The model under review builds one solid part; all positions refer to its coordinate system, in mm. A direction names the side the tool comes from. Give positions to 0.01 mm unless a question says otherwise; leave off trailing zeros. Order: outer loops, then holes, each group sorted by start corner. A loop starts at its lowest first (then second) coordinate and runs counter-clockwise, first axis right, second up. Notation, with made-up numbers: (36, 68.25) -> (90, 68.25) arc R27 ccw to (90, 104.25) -> close; hole circle Ø8 at (15.5, 79). An arc over 180 degrees is marked (long way). Use one line per item in the form item = value.
```python
from build123d import *

# Parameters (mm, degrees)
BASE_FLANGE2_DEPTH         = 3.175
SKETCHED_START             = -176
SKETCHED_BEND3_OUTLINE_W   = 3.175
SKETCHED_BEND3_OUTLINE_H   = 145
SKETCHED_BEND3_DEPTH       = 112.825
SKETCHED_START_2           = 63.175
SKETCHED_BEND3_2_OUTLINE_W = 3.175
SKETCHED_BEND3_2_OUTLINE_H = 145
SKETCHED_BEND3_2_DEPTH     = 112.825
SKETCHED_START_3           = -62.794557784
SKETCHED_BEND3_3_DEPTH     = 2.794557784
SKETCHED_START_4           = 60
SKETCHED_BEND3_4_DEPTH     = 2.794557784
SKETCHED_START_5           = -63.175
SKETCHED_BEND3_5_DEPTH     = 3.9116
SKETCHED_START_6           = 59.2634
SKETCHED_BEND3_6_DEPTH     = 3.9116
SKETCHED_START_7           = -81
SKETCHED_BEND3_7_DEPTH     = 147


with BuildPart() as part:
    # Base-Flange2: sheet metal written as solids
    # Sketch1 → Base-Flange2 (new body)
    with BuildSketch(Plane(origin=(0, 0, 0), x_dir=(1, 0, 0), z_dir=(0, 1, 0))):
        with BuildLine():
            Line((-95, 80), (95, 80))
            Line((95, 80), (138.886329547, 58.22868679))
            ThreePointArc((138.886329547, 58.22868679), (173.284534609, -14.834678268), (110, -65))
            Line((110, -65), (-110, -65))
            ThreePointArc((-110, -65), (-173.284534609, -14.834678268), (-138.886329547, 58.22868679))
            Line((-138.886329547, 58.22868679), (-95, 80))
        make_face()
        with BuildLine():
            Line((100, -15), (120, -15))
            ThreePointArc((120, -15), (123.535533906, -13.535533906), (125, -10))
            Line((125, -10), (125, 10))
            ThreePointArc((125, 10), (123.535533906, 13.535533906), (120, 15))
            Line((120, 15), (100, 15))
            ThreePointArc((100, 15), (96.464466094, 13.535533906), (95, 10))
            Line((95, 10), (95, -10))
            ThreePointArc((95, -10), (96.464466094, -13.535533906), (100, -15))
        make_face(mode=Mode.SUBTRACT)
        with BuildLine():
            Line((-100, -15), (-120, -15))
            ThreePointArc((-120, -15), (-123.535533906, -13.535533906), (-125, -10))
            Line((-125, -10), (-125, 10))
            ThreePointArc((-125, 10), (-123.535533906, 13.535533906), (-120, 15))
            Line((-120, 15), (-100, 15))
            ThreePointArc((-100, 15), (-96.464466094, 13.535533906), (-95, 10))
            Line((-95, 10), (-95, -10))
            ThreePointArc((-95, -10), (-96.464466094, -13.535533906), (-100, -15))
        make_face(mode=Mode.SUBTRACT)
    extrude(amount=-BASE_FLANGE2_DEPTH)

    # Sketched Bend3: read off the stored shape, not the designer's step
    # Sketched Bend3 outline → Sketched Bend3 (cut)
    with BuildSketch(Plane.YZ.offset(SKETCHED_START)):
        with Locations((-1.5875, -7.5)):
            Rectangle(SKETCHED_BEND3_OUTLINE_W, SKETCHED_BEND3_OUTLINE_H)
    extrude(amount=SKETCHED_BEND3_DEPTH, mode=Mode.SUBTRACT)

    # Sketched Bend3 2 outline → Sketched Bend3 2 (cut)
    with BuildSketch(Plane.YZ.offset(SKETCHED_START_2)):
        with Locations((-1.5875, -7.5)):
            Rectangle(SKETCHED_BEND3_2_OUTLINE_W, SKETCHED_BEND3_2_OUTLINE_H)
    extrude(amount=SKETCHED_BEND3_2_DEPTH, mode=Mode.SUBTRACT)

    # Sketched Bend3 3 outline → Sketched Bend3 3 (add)
    with BuildSketch(Plane.YZ.offset(SKETCHED_START_3)):
        with BuildLine():
            Line((47.822512257, 65), (0, 65))
            Line((0, 65), (0, -80))
            Line((0, -80), (32.822512257, -80))
            Line((32.822512257, -80), (76.708841804, -58.22868679))
            ThreePointArc((76.708841804, -58.22868679), (111.107046866, 14.834678268), (47.822512257, 65))
        make_face()
        with BuildLine():
            ThreePointArc((62.822512257, -10), (61.358046163, -13.535533906), (57.822512257, -15))
            Line((57.822512257, -15), (37.822512257, -15))
            ThreePointArc((37.822512257, -15), (34.286978351, -13.535533906), (32.822512257, -10))
            Line((32.822512257, -10), (32.822512257, 10))
            ThreePointArc((32.822512257, 10), (34.286978351, 13.535533906), (37.822512257, 15))
            Line((37.822512257, 15), (57.822512257, 15))
            ThreePointArc((57.822512257, 15), (61.358046163, 13.535533906), (62.822512257, 10))
            Line((62.822512257, 10), (62.822512257, -10))
        make_face(mode=Mode.SUBTRACT)
    extrude(amount=SKETCHED_BEND3_3_DEPTH)

    # Sketched Bend3 4 outline → Sketched Bend3 4 (add)
    with BuildSketch(Plane.YZ.offset(SKETCHED_START_4)):
        with BuildLine():
            Line((47.822512257, 65), (0, 65))
            Line((0, 65), (0, -80))
            Line((0, -80), (32.822512257, -80))
            Line((32.822512257, -80), (76.708841804, -58.22868679))
            ThreePointArc((76.708841804, -58.22868679), (111.107046866, 14.834678268), (47.822512257, 65))
        make_face()
        with BuildLine():
            ThreePointArc((62.822512257, -10), (61.358046163, -13.535533906), (57.822512257, -15))
            Line((57.822512257, -15), (37.822512257, -15))
            ThreePointArc((37.822512257, -15), (34.286978351, -13.535533906), (32.822512257, -10))
            Line((32.822512257, -10), (32.822512257, 10))
            ThreePointArc((32.822512257, 10), (34.286978351, 13.535533906), (37.822512257, 15))
            Line((37.822512257, 15), (57.822512257, 15))
            ThreePointArc((57.822512257, 15), (61.358046163, 13.535533906), (62.822512257, 10))
            Line((62.822512257, 10), (62.822512257, -10))
        make_face(mode=Mode.SUBTRACT)
    extrude(amount=SKETCHED_BEND3_4_DEPTH)

    # Sketched Bend3 5 outline → Sketched Bend3 5 (add)
    with BuildSketch(Plane.YZ.offset(SKETCHED_START_5)):
        with BuildLine():
            ThreePointArc((76.708841804, -58.22868679), (111.107046866, 14.834678268), (47.822512257, 65))
            Line((47.822512257, 65), (0, 65))
            Line((0, 65), (0, -80))
            Line((0, -80), (32.822512257, -80))
            Line((32.822512257, -80), (76.708841804, -58.22868679))
        make_face()
        with BuildLine():
            ThreePointArc((62.822512257, -10), (61.358046163, -13.535533906), (57.822512257, -15))
            Line((57.822512257, -15), (37.822512257, -15))
            ThreePointArc((37.822512257, -15), (34.286978351, -13.535533906), (32.822512257, -10))
            Line((32.822512257, -10), (32.822512257, 10))
            ThreePointArc((32.822512257, 10), (34.286978351, 13.535533906), (37.822512257, 15))
            Line((37.822512257, 15), (57.822512257, 15))
            ThreePointArc((57.822512257, 15), (61.358046163, 13.535533906), (62.822512257, 10))
            Line((62.822512257, 10), (62.822512257, -10))
        make_face(mode=Mode.SUBTRACT)
    extrude(amount=SKETCHED_BEND3_5_DEPTH)

    # Sketched Bend3 6 outline → Sketched Bend3 6 (add)
    with BuildSketch(Plane.YZ.offset(SKETCHED_START_6)):
        with BuildLine():
            ThreePointArc((76.708841804, -58.22868679), (111.107046866, 14.834678268), (47.822512257, 65))
            Line((47.822512257, 65), (0, 65))
            Line((0, 65), (0, -80))
            Line((0, -80), (32.822512257, -80))
            Line((32.822512257, -80), (76.708841804, -58.22868679))
        make_face()
        with BuildLine():
            ThreePointArc((62.822512257, -10), (61.358046163, -13.535533906), (57.822512257, -15))
            Line((57.822512257, -15), (37.822512257, -15))
            ThreePointArc((37.822512257, -15), (34.286978351, -13.535533906), (32.822512257, -10))
            Line((32.822512257, -10), (32.822512257, 10))
            ThreePointArc((32.822512257, 10), (34.286978351, 13.535533906), (37.822512257, 15))
            Line((37.822512257, 15), (57.822512257, 15))
            ThreePointArc((57.822512257, 15), (61.358046163, 13.535533906), (62.822512257, 10))
            Line((62.822512257, 10), (62.822512257, -10))
        make_face(mode=Mode.SUBTRACT)
    extrude(amount=SKETCHED_BEND3_6_DEPTH)

    # Sketched Bend3 7 outline → Sketched Bend3 7 (cut)
    with BuildSketch(Plane.XY.offset(SKETCHED_START_7)):
        with BuildLine():
            Line((-65, -3.175000031), (-59.2634, -3.175))
            ThreePointArc((-59.2634, -3.175), (-62.029318885, -2.029318885), (-63.175, 0.7366))
            Line((-63.175, 0.7366), (-63.175000008, 32.822512257))
            Line((-63.175000008, 32.822512257), (-65, 32.822512257))
            Line((-65, 32.822512257), (-65, -3.175000031))
        make_face()
        with BuildLine():
            ThreePointArc((63.175, 0.7366), (62.029318885, -2.029318885), (59.2634, -3.175))
            Line((59.2634, -3.175), (65, -3.175000031))
            Line((65, -3.175000031), (65, 32.822512257))
            Line((65, 32.822512257), (63.175, 32.822512257))
            Line((63.175, 32.822512257), (63.175, 0.7366))
        make_face()
        with BuildLine():
            Line((-59.2634, 0), (-59.2634, 114))
            Line((-59.2634, 114), (-60, 114))
            Line((-60, 114), (-60, 0.7366))
            ThreePointArc((-60, 0.7366), (-59.784254855, 0.215745145), (-59.2634, 0))
        make_face()
        with BuildLine():
            ThreePointArc((59.2634, 0), (59.784254855, 0.215745145), (60, 0.7366))
            Line((60, 0.7366), (60, 114))
            Line((60, 114), (59.2634, 114))
            Line((59.2634, 114), (59.2634, 0))
        make_face()
    extrude(amount=SKETCHED_BEND3_7_DEPTH, mode=Mode.SUBTRACT)


solid = part.part
```
1. The part is to be moulded in two halves that separate along Y. For faces 4 (the face through (-61.61, 54.458, -69.267)), 5 (the face through (61.565, 61.319, 13.574)), 6 (the face through (-0.3, -0.2, 65)), say which applies: +Y half, -Y half, draft (parallel to the pull), parting line (faces both ways), or undercut.
Values:
face_4 = +Y half
face_5 = undercut
face_6 = draft
2. Add section A-A on y = 17. Give the boundary of the cut face in (x, z) (3 decimals), then the cut area to 3 significant figures.
Values:
outline = (-63.175, -80) -> (-60, -80) -> (-60, 65) -> (-63.175, 65) -> close; (60, -80) -> (63.175, -80) -> (63.175, 65) -> (60, 65) -> close
area = 921 mm^2
3. Add section D-D on x = 30.5. Give the boundary of the cut face in (y, z) (3 decimals).
Values:
outline = (-3.175, -80) -> (0, -80) -> (0, 65) -> (-3.175, 65) -> close
4. For pin 1 Ø1 at (x, z) = (3.5, -15.5) entering from +Y; pin 2 Ø3.5 at (x, z) = (-62, -4.5) entering from -Y; pin 3 Ø2.5 at (x, z) = (-61, 4) entering from +Y, all flat-tipped, find the tip position at first contact; note any pin that passes through.
Values:
pin_1 = 0
pin_2 = -3.05
pin_3 = 112.76
5. Add section C-C on z = -49. Give the boundary of the cut face in (x, y) (3 decimals), then the cut area to 3 significant figures.
Values:
outline = (-63.175, 0.737) arc R3.912 ccw to (-59.263, -3.175) -> (59.263, -3.175) arc R3.912 ccw to (63.175, 0.737) -> (63.175, 90.531) -> (60, 90.531) -> (60, 0.737) arc R0.737 cw to (59.263, 0) -> (-59.263, 0) arc R0.737 cw to (-60, 0.737) -> (-60, 90.531) -> (-63.175, 90.531) -> close
area = 970 mm^2
6. For L1, parallel to X at y = 52.5, z = 22 (3 decimals); L2, parallel to Y at x = 1, z = 19 (3 decimals), list the stretches that pass through material, from the lowest coordinate up.
Values:
L1 = -63.175 to -60, 60 to 63.175
L2 = -3.175 to 0
7. Add section B-B on z = 4. Give the boundary of the cut face in (x, y) (3 decimals), then the cut area to 3 significant figures.
Values:
outline = (-63.175, 0.737) arc R3.912 ccw to (-59.263, -3.175) -> (59.263, -3.175) arc R3.912 ccw to (63.175, 0.737) -> (63.175, 32.823) -> (60, 32.823) -> (60, 0.737) arc R0.737 cw to (59.263, 0) -> (-59.263, 0) arc R0.737 cw to (-60, 0.737) -> (-60, 32.823) -> (-63.175, 32.823) -> close; (-63.175, 62.823) -> (-60, 62.823) -> (-60, 112.699) -> (-63.175, 112.699) -> close; (60, 62.823) -> (63.175, 62.823) -> (63.175, 112.699) -> (60, 112.699) -> close
area = 920 mm^2
8. Tool access review of faces 1 (the face through (61.565, 61.397, -13.496)), 2 (the face through (1, 0, -9)), 3 (the face through (-61.61, 111.374, 13.644)): name each direction out of +Z, -Z, +X, -X, +Y, -Y from which nothing blocks a thin tool from reaching the whole face with its end or side.
Values:
face_1 = +X, -X
face_2 = +Z, -Z, +Y
face_3 = +X, -X, +Y
